Verification items for the finished model (mm, model axes). Face numbers are marked on the shaded views. A direction names the side the tool comes from. Coordinates: 2 decimals unless noted, no trailing zeros. Order: outer loops, then holes, each group sorted by start corner. A loop starts at its lowest first (then second) coordinate and runs counter-clockwise, first axis right, second up. Notation, with made-up numbers: M -20.75,73 L 22.25,73 A27 ccw 22.25,111 Z; hole C 28,62.5 d10. An arc over 180 degrees is marked long. Return JSON: item names as keys, results as strings. Group by question number.
Q1. Section check A-A, the plane x = 0. Enter the section's corners in (y, z), then the cut area to 3 significant figures.
Q2. Section check C-C, the plane y = 0. Count the separate pieces of the cut face and the enclosed holes in it, then the cut area to 3 significant figures.
Q3. Mould release check, pull along Y, two halves, no side actions. Record for the marked faces 1, 2, 3 and 4: pulls with the +Y half, pulls with the -Y half, needs draft (parallel to the pull), parting line crosses it, or undercut.
Q4. Access from +Z, -Z, +X, -X, +Y, -Y to the whole of each face (thin tool, end or side, straight path). Record for the marked faces 5, 6, 7, 8 and 9.
Q5. Section check B-B, the plane z = 12.75. Enter the section's corners in (x, y).
Q6. Thickness scan on probe 1 along X at (y, z) = (-7.5, 22.5); probe 2 along Z at (x, y) = (0, 0); probe 3 along X at (y, z) = (-5, 14.25). Record the ranges inside material, lowest first.
Q7. Go/stop test with flat-tipped pins: pin 1 Ø2.5 at (x, y) = (3, 2) entering from +Z; pin 2 Ø9 at (y, z) = (1.5, 20.5) entering from +X; pin 3 Ø4 at (y, z) = (0, 22) entering from +X; pin 4 Ø13 at (y, z) = (0.5, 24.5) entering from -X. Record where each tip stops, or that it passes through.
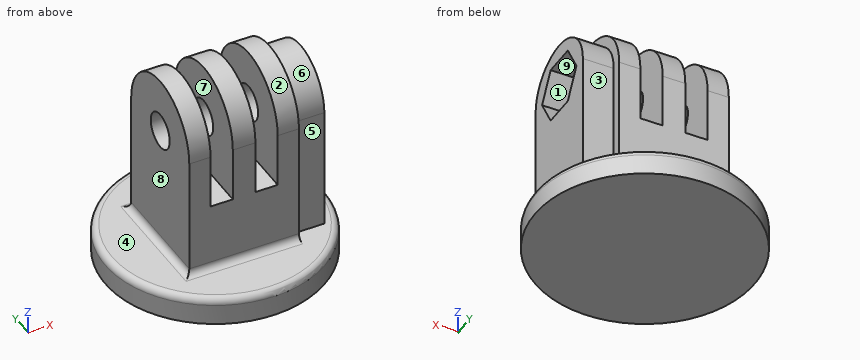
from build123d import *

# Parameters (mm, degrees)
SKETCH_R        = 16
PAD_DEPTH       = 4
FILLET_R        = 1
SKETCH001_W     = 16
SKETCH001_H     = 16
PAD001_DEPTH    = 10
FILLET001_R     = 1
PAD002_DEPTH    = 3.1
PAD003_DEPTH    = 1.65
SKETCH004_R     = 2.6
POCKET_DEPTH    = 24.001
PAD004_DEPTH    = 4.5
POCKET001_DEPTH = 4.5


with BuildPart() as part:
    # Sketch → Pad (new body)
    with BuildSketch(Plane.XY):
        Circle(SKETCH_R)
    extrude(amount=PAD_DEPTH)

    # Fillet
    fillet_edges = [part.edges().sort_by_distance(p)[0] for p in [
        (-16, 0, 4),
    ]]
    fillet(fillet_edges, radius=FILLET_R)

    # Sketch001 (on Face4 of Fillet) → Pad001 (join)
    with BuildSketch(Plane.XY.offset(4)):
        Rectangle(SKETCH001_W, SKETCH001_H)
    extrude(amount=PAD001_DEPTH)

    # Fillet001
    fillet001_edges = [part.edges().sort_by_distance(p)[0] for p in [
        (0, -8, 4),
        (0, 8, 4),
        (-8, 0, 4),
    ]]
    fillet(fillet001_edges, radius=FILLET001_R)

    # Sketch002 (on Face2 of Fillet001) → Pad002 (join)
    with BuildSketch(Plane.YZ.offset(8)):
        with BuildLine():
            Line((-8, 14), (8, 14))
            Line((8, 14), (8, 22))
            ThreePointArc((8, 22), (0, 30), (-8, 22))
            Line((-8, 14), (-8, 22))
        make_face()
    pad002 = extrude(amount=-PAD002_DEPTH)

    # Mirrored: Pad002 across YZ
    add(pad002.mirror(Plane.YZ))

    # Sketch003 → Pad003 (join, symmetric)
    with BuildSketch(Plane.YZ):
        with BuildLine():
            Line((-8, 14), (8, 14))
            Line((8, 14), (8, 22))
            ThreePointArc((8, 22), (0, 30), (-8, 22))
            Line((-8, 14), (-8, 22))
        make_face()
    extrude(amount=PAD003_DEPTH, both=True)

    # Sketch004 (on Face8 of Pad003) → Pocket (cut, through all)
    with BuildSketch(Plane.YZ.offset(8)):
        with Locations((0, 22)):
            Circle(SKETCH004_R)
    extrude(amount=-POCKET_DEPTH, mode=Mode.SUBTRACT)

    # Sketch005 (on Face8 of Pocket) → Pad004 (join)
    with BuildSketch(Plane.YZ.offset(8)):
        with BuildLine():
            Line((-6.5, 4), (-6.5, 22))
            ThreePointArc((6.5, 22), (0, 28.5), (-6.5, 22))
            Line((6.5, 4), (6.5, 22))
            Line((-6.5, 4), (6.5, 4))
        make_face()
    extrude(amount=PAD004_DEPTH)

    # Sketch006 (on Face5 of Pad004) → Pocket001 (cut)
    with BuildSketch(Plane.YZ.offset(12.5)):
        Polygon((2.367136, 26.1), (-2.367136, 26.1), (-4.734272, 22), (-2.367136, 17.9), (2.367136, 17.9), (4.734272, 22), align=None)
    extrude(amount=-POCKET001_DEPTH, mode=Mode.SUBTRACT)


solid = part.part
Numbers:
{
 "1": {"outline": "M -16,0 L 16,0 L 16,3 A1 ccw 15,4 L 9,4 A1 cw 8,5 L 8,22 A8 ccw -8,22 L -8,5 A1 cw -9,4 L -15,4 A1 ccw -16,3 Z; hole C 0,22 d5.2", "area": "495 mm2"},
 "2": {"separate pieces": "4", "enclosed holes": "0", "area": "464 mm2"},
 "3": {"face 1": "undercut", "face 2": "parting line crosses it", "face 3": "pulls with the +Y half", "face 4": "needs draft"},
 "4": {"face 5": "+Z, +X, -Y", "face 6": "+Z, +X", "face 7": "+Z, +Y, -Y", "face 8": "+Z, -X, +Y, -Y", "face 9": "+X"},
 "5": {"outline": "M -8,-8 L 8,-8 L 8,-6.5 L 12.5,-6.5 L 12.5,6.5 L 8,6.5 L 8,8 L -8,8 Z"},
 "6": {"probe 1": "x = -8 to -4.9, -1.65 to 1.65, 4.9 to 8", "probe 2": "z = 0 to 19.4, 24.6 to 30", "probe 3": "x = -8 to -4.9, -1.65 to 1.65, 4.9 to 12.5"},
 "7": {"pin 1": "stops at z = 14", "pin 2": "stops at x = 12.5", "pin 3": "passes through", "pin 4": "stops at x = -8"}
}
